from build123d import *

# Parameters (mm, degrees)
F0_R     = 0.5
F1_DEPTH = 5
F2_R     = 1.25
F3_DEPTH = 2.5


# Not quite as in the source:
# - a fillet or chamfer that OpenCascade refuses, or shapes differently, is made with other operations: its cross-section is extruded or revolved along the edge and cut away or added


with BuildPart() as f1:
    # F0 (on Top) → F1 (new body)
    with BuildSketch(Plane.XY):
        Circle(F0_R)
    extrude(amount=F1_DEPTH)

    # F2 (on face) → F3 (join)
    with BuildSketch(Plane.XY.offset(5)):
        Circle(F2_R)
    extrude(amount=F3_DEPTH)

    # F4: fillet of radius 1.2 on 2 edges, made by hand

    # F4_s1 → F4_t2 (revolve, cut)
    with BuildSketch(Plane.XZ):
        with BuildLine():
            ThreePointArc((1.25, 6.3), (0.8985281374, 7.1485281374), (0.05, 7.5))
            Line((0.05, 7.5), (1.25, 7.5))
            Line((1.25, 7.5), (1.25, 6.3))
        make_face()
    revolve(axis=Axis((0, 0, 7.5), (0, 0, 1)), mode=Mode.SUBTRACT)

    # F4_s3 → F4_t4 (revolve, cut)
    with BuildSketch(Plane.XZ):
        with BuildLine():
            ThreePointArc((1.25, 6.1124297731), (1.0449874371, 5.4416093798), (0.5, 5))
            Line((0.5, 5), (1.25, 5))
            Line((1.25, 5), (1.25, 6.1124297731))
        make_face()
    revolve(axis=Axis((0, 0, 5), (0, 0, 1)), mode=Mode.SUBTRACT)


solid = f1.part
Build history of the part. All positions in model axes, mm. A direction names the side the tool comes from. Coordinates: 2 decimals unless noted, no trailing zeros. Order: outer loops, then holes, each group sorted by start corner. A loop starts at its lowest first (then second) coordinate and runs counter-clockwise, first axis right, second up. Notation, with made-up numbers: (11.5, 48) -> (59.5, 48) arc R29 cw to (59.5, 72) -> close; hole circle Ø1 at (5, 73). An arc over 180 degrees is marked (long way). One line per item, written item: value.
(1) Slice it at A-A, the plane z = 2.25. List the corners of the cut face in (x, y).
Checked values:
outline: circle Ø1 at (0, 0)
(2) Drop a flat-ended pin along its axis: pin 1 Ø1 at (x, y) = (1, 0.5) entering from -Z. Give the stop position or say it passes through.
Checked values:
pin 1: z = 5.06
(3) Probe line 1 (X direction, y = 0.5, z = 5.5); line 2 (Z direction, x = 0, y = -0.8); line 3 (Z direction, x = -0.4, y = 0.6). List the from-to ranges inside material, lowest first. Write a range as [from, to].
Checked values:
line 1: [-0.96, 0.96]
line 2: [5.18, 7.24]
line 3: [5.12, 7.29]
(4) Tool access for faces 1 (the cylindrical face through (-0.108, -0.488, 2.465)), 2 (the flat face through (0, 0, 0)): list every direction of +Z, -Z, +X, -X, +Y, -Y with a clear straight run to the whole face (end or side of a thin tool).
Checked values:
face 1: -Z
face 2: -Z, +X, -X, +Y, -Y
